from build123d import *

# Parameters (mm, degrees)
F0_W     = 1000
F0_H     = 2000
F1_DEPTH = 1500
F2_W     = 800
F2_H     = 400
F3_DEPTH = 2000
F4_W     = 1800
F4_H     = 400
F5_DEPTH = 1000


with BuildPart() as f1:
    # F0 (on Top) → F1 (new body)
    with BuildSketch(Plane.XY):
        with Locations((-500, 1000)):
            Rectangle(F0_W, F0_H)
    extrude(amount=F1_DEPTH)

    # F2 (on face) → F3 (cut)
    with BuildSketch(Plane.XZ):
        with Locations((-500, 200)):
            Rectangle(F2_W, F2_H)
    extrude(amount=-F3_DEPTH, mode=Mode.SUBTRACT)

    # F4 (on face) → F5 (cut)
    with BuildSketch(Plane.YZ):
        with Locations((1000, 200)):
            Rectangle(F4_W, F4_H)
    extrude(amount=-F5_DEPTH, mode=Mode.SUBTRACT)


solid = f1.part
Work out the finished part from the listing and answer in its coordinate system (mm). A direction names the side the tool comes from. Round coordinates to 2 decimals unless told otherwise and drop trailing zeros. Write each loop counter-clockwise with the first axis right and the second up, starting at its lowest first coordinate (ties: lowest second). Pieces come first, ordered by that corner, then holes. Notation, with made-up numbers: (18, 2) - (22, 2) arc R18 ccw to (22, 9) - close; hole circle Ø11 at (71.25, 49). An arc over 180 degrees is marked (long way). Answer in a Markdown table with one row per item. Add a question column.
1. A cutting plane is placed at A-A, the plane z = 247.5. Determine the outline of the cut face in (x, y).
2. Find the intervals of material crossed by line 1 along Y through (x, z) = (-918, 112); line 2 along Z through (x, y) = (-420, 357), in increasing order. Write a range as from..to.
3. A cutting plane is placed at B-B, the plane y = 1319. Determine the outline of the cut face in (x, z), and give its area (3 significant figures).
4. The mould has two halves that part along Y. Classify faces 4 (the flat face through (-949, 100, 197)), 5 (the flat face through (-951, 51, 0)), 6 (the flat face through (-493, 986, 400)), 7 (the flat face through (-507, 2000, 906)): +Y half, -Y half, draft (parallel to the pull), parting line (faces both ways), or undercut.
5. A cutting plane is placed at C-C, the plane x = -365. Determine the outline of the cut face in (y, z), and give its area (3 significant figures).
6. For faces 1 (the flat face through (-49, 1900, 197)), 2 (the flat face through (0, 986, 906)), 3 (the flat face through (-100, 1949, 197)), determine the directions among +Z, -Z, +X, -X, +Y, -Y from which every point of the face is accessible in a straight line to the end or side of a thin tool.
7. Given pin 1 (2 mm diameter, centred on x = -642, z = 1116, fed in from -Y); pin 2 (6 mm diameter, centred on x = -477, y = 1242.5, fed in from -Z), each flat-ended and moving along its own axis, determine where each tip first touches the part or whether it passes through.
Worked out:
| question | item | result |
|---|---|---|
| 1 | outline | (-1000, 0) - (-900, 0) - (-900, 100) - (-1000, 100) - close; (-1000, 1900) - (-900, 1900) - (-900, 2000) - (-1000, 2000) - close; (-100, 0) - (0, 0) - (0, 100) - (-100, 100) - close; (-100, 1900) - (0, 1900) - (0, 2000) - (-100, 2000) - close |
| 2 | line 1 | 0..100, 1900..2000 |
| 2 | line 2 | 400..1500 |
| 3 | outline | (-1000, 400) - (0, 400) - (0, 1500) - (-1000, 1500) - close |
| 3 | area | 1,100,000 mm^2 |
| 4 | face 4 | undercut |
| 4 | face 5 | draft |
| 4 | face 6 | undercut |
| 4 | face 7 | +Y half |
| 5 | outline | (0, 400) - (2000, 400) - (2000, 1500) - (0, 1500) - close |
| 5 | area | 2,200,000 mm^2 |
| 6 | face 1 | -Z, +X, -X |
| 6 | face 2 | +Z, -Z, +X, +Y, -Y |
| 6 | face 3 | -Z, +Y, -Y |
| 7 | pin 1 | y = 0 |
| 7 | pin 2 | z = 400 |
